Could you check a few things on this model? Use its own coordinates, in mm. Coordinates: 2 decimals unless noted, no trailing zeros. Order: outer loops, then holes, each group sorted by start corner. A loop starts at its lowest first (then second) coordinate and runs counter-clockwise, first axis right, second up. Notation, with made-up numbers: (-36.75, 24.25) - (3.25, 24.25) arc R28 ccw to (3.25, 46.25) - close; hole circle Ø1 at (-27, 68.25). An arc over 180 degrees is marked (long way). Answer as a JSON object with one key per item and string values. Group by question number.
(1) Will these pins go through, and if not, where does the flat tip stop? P1, Ø1, axis at y = 11.5, z = 20, coming from the +X side (3 decimals); P2, Ø3, axis at x = 77, y = 10, coming from the -Z side; P3, Ø10, axis at x = 95.25, z = 31.75, coming from the +Y side.
(2) Imagine slicing it at D-D, the plane z = 13. Write out the boundary of the cut face in (x, y).
(3) Please list where these lines run through material, in increasing order: probe 1 along X at (y, z) = (8.5, 31.75); probe 2 along X at (y, z) = (3.25, 5.5) (3 decimals); probe 3 along Z at (x, y) = (81, 5).
(4) Imagine slicing it at B-B, the plane y = 9.25. Give the number of separate pieces and of enclosed holes in the cut face, and give its area (3 significant figures).
(5) Imagine slicing it at A-A, the plane z = 31.75. Write out the boundary of the cut face in (x, y).
(6) Imagine slicing it at C-C, the plane x = 95.25. Write out the boundary of the cut face in (y, z).
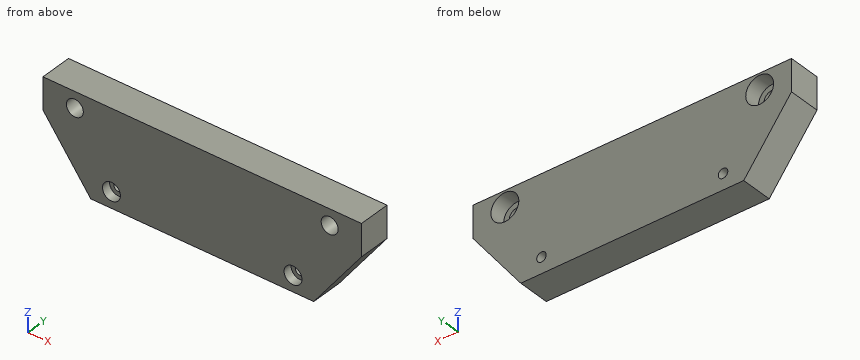
from build123d import *

# Parameters (mm, degrees)
BOSS_EXTRUDE3_DEPTH                              = 12.7
CBORE_FOR_6_SOCKET_HEAD_CAP_SCREW1_D             = 3.7973
CBORE_FOR_6_SOCKET_HEAD_CAP_SCREW1_CBORE_D       = 7.14502
CBORE_FOR_6_SOCKET_HEAD_CAP_SCREW1_CBORE_DEPTH   = 3.5052
CBORE_FOR_1_4_SOCKET_HEAD_CAP_SCREW1_D           = 6.7564
CBORE_FOR_1_4_SOCKET_HEAD_CAP_SCREW1_CBORE_D     = 11.1125
CBORE_FOR_1_4_SOCKET_HEAD_CAP_SCREW1_CBORE_DEPTH = 6.35


with BuildPart() as part:
    # Sketch8 → Boss-Extrude3 (new body)
    with BuildSketch(Plane(origin=(0, 0, 0), x_dir=(1, 0, 0), z_dir=(0, 1, 0))):
        Polygon((0, 0), (88.9, 0), (107.95, -25.4), (107.95, -38.1), (-19.05, -38.1), (-19.05, -25.4), align=None)
    extrude(amount=BOSS_EXTRUDE3_DEPTH)

    # CBORE for #6 Socket Head Cap Screw1 (through all)
    with Locations(Plane(origin=(0, 0, 0), x_dir=(-1, 0, 0), z_dir=(0, -1, 0))):
        with Locations((-80.645, -6.35), (-8.255, -6.35)):
            CounterBoreHole(CBORE_FOR_6_SOCKET_HEAD_CAP_SCREW1_D / 2, CBORE_FOR_6_SOCKET_HEAD_CAP_SCREW1_CBORE_D / 2, CBORE_FOR_6_SOCKET_HEAD_CAP_SCREW1_CBORE_DEPTH)

    # CBORE for 1/4 Socket Head Cap Screw1 (through all)
    with Locations(Plane(origin=(0, 12.7, 0), x_dir=(1, 0, 0), z_dir=(0, 1, 0))):
        with Locations((-6.35, -31.75), (95.25, -31.75)):
            CounterBoreHole(CBORE_FOR_1_4_SOCKET_HEAD_CAP_SCREW1_D / 2, CBORE_FOR_1_4_SOCKET_HEAD_CAP_SCREW1_CBORE_D / 2, CBORE_FOR_1_4_SOCKET_HEAD_CAP_SCREW1_CBORE_DEPTH)


solid = part.part
Result set:
{
 "1": {"P1": "stops at x = 104.275", "P2": "stops at z = 0", "P3": "stops at y = 6.35"},
 "2": {"outline": "(-9.75, 0) - (98.65, 0) - (98.65, 12.7) - (-9.75, 12.7) - close"},
 "3": {"probe 1": "x = -19.05 to -11.91, -0.79 to 89.69, 100.81 to 107.95", "probe 2": "x = -4.125 to 4.785, 11.725 to 77.175, 84.115 to 93.025", "probe 3": "z = 0 to 4.48, 8.22 to 38.1"},
 "4": {"separate pieces": "1", "enclosed holes": "4", "area": "4,140 mm^2"},
 "5": {"outline": "(-19.05, 0) - (-9.73, 0) - (-9.73, 6.35) - (-11.91, 6.35) - (-11.91, 12.7) - (-19.05, 12.7) - close; (-2.97, 0) - (91.87, 0) - (91.87, 6.35) - (89.69, 6.35) - (89.69, 12.7) - (-0.79, 12.7) - (-0.79, 6.35) - (-2.97, 6.35) - close; (98.63, 0) - (107.95, 0) - (107.95, 12.7) - (100.81, 12.7) - (100.81, 6.35) - (98.63, 6.35) - close"},
 "6": {"outline": "(0, 8.47) - (12.7, 8.47) - (12.7, 26.19) - (6.35, 26.19) - (6.35, 28.37) - (0, 28.37) - close; (0, 35.13) - (6.35, 35.13) - (6.35, 37.31) - (12.7, 37.31) - (12.7, 38.1) - (0, 38.1) - close"}
}
